```python
from build123d import *

# Parameters (mm, degrees)
SKETCH1_W               = 10
SKETCH1_H               = 19.05
BOSS_EXTRUDE1_DEPTH     = 1
SKETCH2_W               = 0.5
SKETCH2_H               = 15
CUT_EXTRUDE1_DEPTH      = 1
CUT_EXTRUDE1_DEPTH_BACK = 2
SKETCH3_W               = 0.5
SKETCH3_H               = 15
CUT_EXTRUDE2_DEPTH      = 2
SKETCH4_W               = 5
SKETCH4_H               = 2
CUT_EXTRUDE3_DEPTH      = 2
SKETCH5_W               = 5
SKETCH5_H               = 13
CUT_EXTRUDE4_DEPTH      = 0.5
FILLET9_R               = 0.25
FILLET10_R              = 0.25
FILLET11_R              = 0.25
FILLET13_R              = 1
FILLET14_R              = 1
FILLET15_R              = 1
FILLET16_R              = 1


with BuildPart() as part:
    # Sketch1 → Boss-Extrude1 (new body)
    with BuildSketch(Plane(origin=(0, 0, 0), x_dir=(1, 0, 0), z_dir=(0, 1, 0))):
        Rectangle(SKETCH1_W, SKETCH1_H)
    extrude(amount=BOSS_EXTRUDE1_DEPTH)

    # Sketch2 → Cut-Extrude1 (cut, two sides)
    with BuildSketch(Plane(origin=(0, 1, 0), x_dir=(1, 0, 0), z_dir=(0, 1, 0))) as cut_extrude1_sk:
        with Locations((-2.75, 0.025)):
            Rectangle(SKETCH2_W, SKETCH2_H)
    extrude(amount=CUT_EXTRUDE1_DEPTH, mode=Mode.SUBTRACT)
    extrude(cut_extrude1_sk.sketch, amount=-CUT_EXTRUDE1_DEPTH_BACK, mode=Mode.SUBTRACT)

    # Sketch3 → Cut-Extrude2 (cut, through all)
    with BuildSketch(Plane(origin=(0, 1, 0), x_dir=(1, 0, 0), z_dir=(0, 1, 0))):
        with Locations((2.75, 0.025)):
            Rectangle(SKETCH3_W, SKETCH3_H)
    extrude(amount=-CUT_EXTRUDE2_DEPTH, mode=Mode.SUBTRACT)

    # Sketch4 → Cut-Extrude3 (cut, through all)
    with BuildSketch(Plane(origin=(0, 1, 0), x_dir=(1, 0, 0), z_dir=(0, 1, 0))):
        with Locations((0, 6.525)):
            Rectangle(SKETCH4_W, SKETCH4_H)
    extrude(amount=-CUT_EXTRUDE3_DEPTH, mode=Mode.SUBTRACT)

    # Sketch5 → Cut-Extrude4 (cut)
    with BuildSketch(Plane(origin=(0, 1, 0), x_dir=(1, 0, 0), z_dir=(0, 1, 0))):
        with Locations((0, -0.975)):
            Rectangle(SKETCH5_W, SKETCH5_H)
    extrude(amount=-CUT_EXTRUDE4_DEPTH, mode=Mode.SUBTRACT)

    # Fillet9
    fillet9_edges = [part.edges().sort_by_distance(p)[0] for p in [
        (0, 0.5, -5.525),
    ]]
    fillet(fillet9_edges, radius=FILLET9_R)

    # Fillet10
    fillet10_edges = [part.edges().sort_by_distance(p)[0] for p in [
        (-2.5, 0.125, -5.525),
        (-2.5, 0.5, 1.1),
    ]]
    fillet(fillet10_edges, radius=FILLET10_R)

    # Fillet11
    fillet11_edges = [part.edges().sort_by_distance(p)[0] for p in [
        (2.5, 0.125, -5.525),
        (2.5, 0.5, 1.1),
    ]]
    fillet(fillet11_edges, radius=FILLET11_R)

    # Fillet13
    fillet13_edges = [part.edges().sort_by_distance(p)[0] for p in [
        (-5, 0.5, -9.525),
    ]]
    fillet(fillet13_edges, radius=FILLET13_R)

    # Fillet14
    fillet14_edges = [part.edges().sort_by_distance(p)[0] for p in [
        (5, 0.5, -9.525),
    ]]
    fillet(fillet14_edges, radius=FILLET14_R)

    # Fillet15
    fillet15_edges = [part.edges().sort_by_distance(p)[0] for p in [
        (5, 0.5, 9.525),
    ]]
    fillet(fillet15_edges, radius=FILLET15_R)

    # Fillet16
    fillet16_edges = [part.edges().sort_by_distance(p)[0] for p in [
        (-5, 0.5, 9.525),
    ]]
    fillet(fillet16_edges, radius=FILLET16_R)


solid = part.part
```
Input: part model. Units: mm. Frame: model coordinates. A direction names the side the tool comes from. Give positions to 0.01 mm unless a question says otherwise; leave off trailing zeros. Loops run counter-clockwise (first coordinate to the right, second up) from the corner with the lowest first, then second, coordinate; pieces in that order, holes last.
1) Contact query for a flat-ended pin moving along its axis: pin 1 (3.5 mm diameter, centred on x = -1, z = 2.5, fed in from +Y). Output: stop coordinate, or through.
A:
pin 1: stops at y = 0.5
2) Line query: L1, parallel to X at y = 0.2, z = 3.5; L2, parallel to Z at x = 1.75, y = 0.65 (3 decimals); L3, parallel to X at y = 0.65, z = 4.5. Output: solid intervals per line, ascending.
A:
L1: x = -5 to -3, -2.5 to 2.5, 3 to 5
L2: z = -9.525 to -7.525, 7.475 to 9.525
L3: x = -5 to -3, 3 to 5
3) Reachability of faces 4 (the flat face through (0, 0.5, -7.525)), 5 (the cylindrical face through (4.715, 0.507, 9.224)), 6 (the flat face through (0, 0.5, 1)) from +Z, -Z, +X, -X, +Y, -Y: full face, straight path, thin tool, end or side. Return the list, or none.
A:
face 4: +Y, -Y
face 5: +Z, +X, +Y, -Y
face 6: +Y
4) Section query A-A on x = 0. Return the cut outline in (y, z) (3 decimals), and give its area (3 significant figures).
A:
outline: (0, -9.525) - (1, -9.525) - (1, -7.525) - (0, -7.525) - close; (0, -5.525) - (0.25, -5.525) arc R0.25 ccw to (0.5, -5.275) - (0.5, 7.475) - (1, 7.475) - (1, 9.525) - (0, 9.525) - close
area: 10.5 mm2
5) Section query D-D on z = 6. Return the cut outline in (x, y).
A:
outline: (-5, 0) - (-3, 0) - (-3, 1) - (-5, 1) - close; (-2.5, 0) - (2.5, 0) - (2.5, 0.25) arc R0.25 ccw to (2.25, 0.5) - (-2.25, 0.5) arc R0.25 ccw to (-2.5, 0.25) - close; (3, 0) - (5, 0) - (5, 1) - (3, 1) - close
6) Section query C-C on z = -7. Return the cut outline in (x, y), and give its area (3 significant figures).
A:
outline: (-5, 0) - (-3, 0) - (-3, 1) - (-5, 1) - close; (3, 0) - (5, 0) - (5, 1) - (3, 1) - close
area: 4.00 mm2
7) Section query B-B on y = 0.7. Return the cut outline in (x, z) (3 decimals), and give its area (3 significant figures).
A:
outline: (-5, -8.525) arc R1 ccw to (-4, -9.525) - (4, -9.525) arc R1 ccw to (5, -8.525) - (5, 8.525) arc R1 ccw to (4, 9.525) - (-4, 9.525) arc R1 ccw to (-5, 8.525) - close; hole (-3, -7.525) - (3, -7.525) - (3, 7.475) - (-3, 7.475) - close
area: 99.6 mm2
8) Mould query, pull axis X, two halves, no side actions, for faces 1 (the cylindrical face through (-4.7, 0.51, 9.24)), 2 (the flat face through (-3, 0.5, 0.1)), 3 (the flat face through (-0.1, 0.5, -9.525)). Classes: released by +X, released by -X, zero draft, split by the parting line, or undercut.
A:
face 1: released by -X
face 2: undercut
face 3: zero draft
